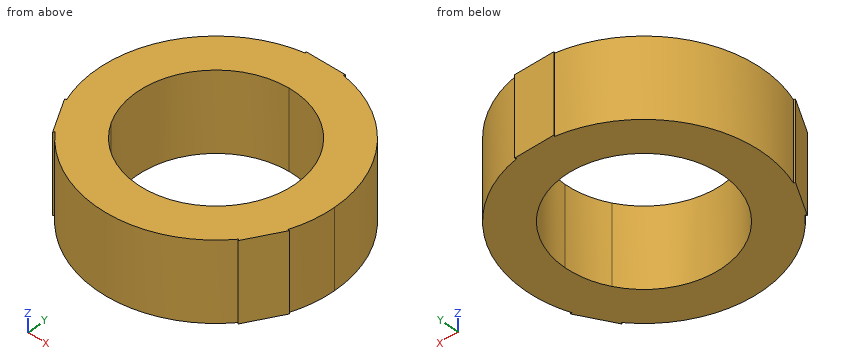
from build123d import *

# Parameters (mm, degrees)
F1_DEPTH = 12.7


with BuildPart() as f1:
    # F0 (on Top) → F1 (new body)
    with BuildSketch(Plane.XY):
        with BuildLine():
            ThreePointArc((0, 12.7), (8.9802561211, 8.9802561211), (12.7, 0))
            ThreePointArc((12.7, 0), (12.2672579939, -3.2870018728), (10.9985226281, -6.35))
            Line((10.9985226281, -6.35), (17.8106697795, -6.7588861512))
            ThreePointArc((17.8106697795, -6.7588861512), (18.7376060277, -3.4357852596), (19.05, 0))
            ThreePointArc((19.05, 0), (14.5093501963, 12.3442803306), (3.0519677815, 18.8039355631))
            Line((3.0519677815, 18.8039355631), (0, 12.7))
        make_face()
        with BuildLine():
            Line((-3.0519677815, 18.8039355631), (0, 12.7))
            Line((0, 12.7), (0, 19.05))
            ThreePointArc((0, 19.05), (-1.5309355838, 18.9883842451), (-3.0519677815, 18.8039355631))
        make_face()
        with BuildLine():
            ThreePointArc((-10.9985226281, -6.35), (-10.9985226281, 6.35), (0, 12.7))
            Line((0, 12.7), (-3.0519677815, 18.8039355631))
            ThreePointArc((-3.0519677815, 18.8039355631), (-16.4977839421, 9.525), (-17.8106697795, -6.7588861512))
            Line((-17.8106697795, -6.7588861512), (-10.9985226281, -6.35))
        make_face()
        with BuildLine():
            Line((0, 19.05), (0, 12.7))
            Line((0, 12.7), (3.0519677815, 18.8039355631))
            ThreePointArc((3.0519677815, 18.8039355631), (1.5309355838, 18.9883842451), (0, 19.05))
        make_face()
        with BuildLine():
            Line((14.758701998, -12.0450494119), (10.9985226281, -6.35))
            ThreePointArc((10.9985226281, -6.35), (0, -12.7), (-10.9985226281, -6.35))
            Line((-10.9985226281, -6.35), (-14.758701998, -12.0450494119))
            ThreePointArc((-14.758701998, -12.0450494119), (0, -19.05), (14.758701998, -12.0450494119))
        make_face()
        with BuildLine():
            Line((17.8106697795, -6.7588861512), (10.9985226281, -6.35))
            Line((10.9985226281, -6.35), (16.4977839421, -9.525))
            ThreePointArc((16.4977839421, -9.525), (17.2098909249, -8.1683630154), (17.8106697795, -6.7588861512))
        make_face()
        with BuildLine():
            Line((16.4977839421, -9.525), (10.9985226281, -6.35))
            Line((10.9985226281, -6.35), (14.758701998, -12.0450494119))
            ThreePointArc((14.758701998, -12.0450494119), (15.6789553412, -10.8200212296), (16.4977839421, -9.525))
        make_face()
        with BuildLine():
            Line((-14.758701998, -12.0450494119), (-10.9985226281, -6.35))
            Line((-10.9985226281, -6.35), (-16.4977839421, -9.525))
            ThreePointArc((-16.4977839421, -9.525), (-15.6789553412, -10.8200212296), (-14.758701998, -12.0450494119))
        make_face()
        with BuildLine():
            Line((-16.4977839421, -9.525), (-10.9985226281, -6.35))
            Line((-10.9985226281, -6.35), (-17.8106697795, -6.7588861512))
            ThreePointArc((-17.8106697795, -6.7588861512), (-17.2098909249, -8.1683630154), (-16.4977839421, -9.525))
        make_face()
        with BuildLine():
            Line((3.175, 19.05), (0, 19.05))
            ThreePointArc((0, 19.05), (1.5309355838, 18.9883842451), (3.0519677815, 18.8039355631))
            Line((3.0519677815, 18.8039355631), (3.175, 19.05))
        make_face()
        with BuildLine():
            ThreePointArc((-3.0519677815, 18.8039355631), (-1.5309355838, 18.9883842451), (0, 19.05))
            Line((0, 19.05), (-3.175, 19.05))
            Line((-3.175, 19.05), (-3.0519677815, 18.8039355631))
        make_face()
        with BuildLine():
            Line((14.9102839421, -12.274630657), (16.4977839421, -9.525))
            ThreePointArc((16.4977839421, -9.525), (15.6789553412, -10.8200212296), (14.758701998, -12.0450494119))
            Line((14.758701998, -12.0450494119), (14.9102839421, -12.274630657))
        make_face()
        with BuildLine():
            ThreePointArc((17.8106697795, -6.7588861512), (17.2098909249, -8.1683630154), (16.4977839421, -9.525))
            Line((16.4977839421, -9.525), (18.0852839421, -6.775369343))
            Line((18.0852839421, -6.775369343), (17.8106697795, -6.7588861512))
        make_face()
        with BuildLine():
            Line((-18.0852839421, -6.775369343), (-16.4977839421, -9.525))
            ThreePointArc((-16.4977839421, -9.525), (-17.2098909249, -8.1683630154), (-17.8106697795, -6.7588861512))
            Line((-17.8106697795, -6.7588861512), (-18.0852839421, -6.775369343))
        make_face()
        with BuildLine():
            ThreePointArc((-14.758701998, -12.0450494119), (-15.6789553412, -10.8200212296), (-16.4977839421, -9.525))
            Line((-16.4977839421, -9.525), (-14.9102839421, -12.274630657))
            Line((-14.9102839421, -12.274630657), (-14.758701998, -12.0450494119))
        make_face()
    extrude(amount=F1_DEPTH)


solid = f1.part
Geometry check sheet. Reference: the model listing, model coordinates, mm. Round coordinates to 2 decimals unless told otherwise and drop trailing zeros. Write each loop counter-clockwise with the first axis right and the second up, starting at its lowest first coordinate (ties: lowest second). Pieces come first, ordered by that corner, then holes. Notation, with made-up numbers: (-12.75, 70) - (14.25, 70) arc R24 ccw to (14.25, 88) - close; hole circle Ø11 at (-3, 80.25). An arc over 180 degrees is marked (long way). One line per item, written item: value.
1. Depth check by flat-ended pin: pin 1 Ø1.5 at (y, z) = (7.5, 2.5) entering from +X; pin 2 Ø2 at (x, z) = (-13, 4) entering from -Y; pin 3 Ø6 at (x, y) = (-1, 10.5) entering from -Z; pin 4 Ø2 at (y, z) = (7.5, 11) entering from -X. Enter the tip coordinate at first touch or a pass-through.
The answers:
pin 1: stops at x = 17.81
pin 2: stops at y = -14.8
pin 3: stops at z = 0
pin 4: stops at x = -17.91
2. Cross-section at A-A on z = 3.5. Record the boundary of the cut face in (x, y) (3 decimals).
The answers:
outline: (-18.085, -6.775) - (-14.91, -12.275) - (-14.759, -12.045) arc R19.05 ccw to (14.759, -12.045) - (14.91, -12.275) - (18.085, -6.775) - (17.811, -6.759) arc R19.05 ccw to (3.052, 18.804) - (3.175, 19.05) - (-3.175, 19.05) - (-3.052, 18.804) arc R19.05 ccw to (-17.811, -6.759) - close; hole circle Ø25.4 at (0, 0)
3. Cross-section at C-C on y = -7.5. Record the boundary of the cut face in (x, z), and give its area (3 significant figures).
The answers:
outline: (-17.67, 0) - (-10.25, 0) - (-10.25, 12.7) - (-17.67, 12.7) - close; (10.25, 0) - (17.67, 0) - (17.67, 12.7) - (10.25, 12.7) - close
area: 188 mm^2
4. Scan lines: L1, parallel to X at y = -0.5, z = 11.75; L2, parallel to Y at x = 0.5, z = 1; L3, parallel to X at y = -5, z = 11. Record each from-to range of solid material in increasing order.
The answers:
L1: x = -19.04 to -12.69, 12.69 to 19.04
L2: y = -19.04 to -12.69, 12.69 to 19.05
L3: x = -18.38 to -11.67, 11.67 to 18.38
5. Cross-section at B-B on x = 5.5. Record the boundary of the cut face in (y, z).
The answers:
outline: (-18.24, 0) - (-11.45, 0) - (-11.45, 12.7) - (-18.24, 12.7) - close; (11.45, 0) - (18.24, 0) - (18.24, 12.7) - (11.45, 12.7) - close
6. Cross-section at D-D on x = 16. Record the boundary of the cut face in (y, z).
The answers:
outline: (-10.39, 0) - (10.34, 0) - (10.34, 12.7) - (-10.39, 12.7) - close
